Geometry: final body of the model. Coordinates: model frame, mm. Round coordinates to 2 decimals unless told otherwise and drop trailing zeros. Write each loop counter-clockwise with the first axis right and the second up, starting at its lowest first coordinate (ties: lowest second). Pieces come first, ordered by that corner, then holes. Notation, with made-up numbers: (34.25, 79) - (59.25, 79) arc R13 ccw to (59.25, 96) - close; hole circle Ø10 at (68.5, 13.5). An arc over 180 degrees is marked (long way). Write each question's results on one line, items separated by ' | '.
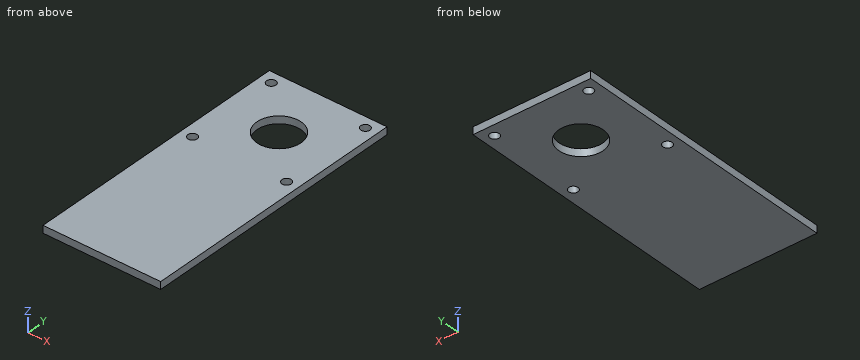
from build123d import *

# Parameters (mm, degrees)
SKETCH2_W           = 50.8
SKETCH2_H           = 50.8
SKETCH2_R           = 2
SKETCH2_R_2         = 9.525
BOSS_EXTRUDE1_DEPTH = 3.175
SKETCH3_W           = 50.8
SKETCH3_H           = 3.175
BOSS_EXTRUDE2_DEPTH = 66.04


with BuildPart() as part:
    # Sketch2 → Boss-Extrude1 (new body)
    with BuildSketch(Plane.XY):
        with Locations((25.4, 25.4)):
            Rectangle(SKETCH2_W, SKETCH2_H)
        with Locations((5.08, 45.72)):
            Circle(SKETCH2_R, mode=Mode.SUBTRACT)
        with Locations((45.72, 45.72)):
            Circle(SKETCH2_R, mode=Mode.SUBTRACT)
        with Locations((45.72, 5.08)):
            Circle(SKETCH2_R, mode=Mode.SUBTRACT)
        with Locations((5.08, 5.08)):
            Circle(SKETCH2_R, mode=Mode.SUBTRACT)
        with Locations((25.4, 25.4)):
            Circle(SKETCH2_R_2, mode=Mode.SUBTRACT)
    extrude(amount=BOSS_EXTRUDE1_DEPTH)

    # Sketch3 → Boss-Extrude2 (add)
    with BuildSketch(Plane.XZ):
        with Locations((25.4, 1.5875)):
            Rectangle(SKETCH3_W, SKETCH3_H)
    extrude(amount=BOSS_EXTRUDE2_DEPTH)


solid = part.part
Q1. Section query B-B, the plane z = 1.8. Return loops of the section in (x, y) (3 decimals).
Answer block:
outline: (0, -66.04) - (50.8, -66.04) - (50.8, 50.8) - (0, 50.8) - close; hole circle Ø4 at (5.08, 5.08); hole circle Ø4 at (5.08, 45.72); hole circle Ø19.05 at (25.4, 25.4); hole circle Ø4 at (45.72, 5.08); hole circle Ø4 at (45.72, 45.72)
Q2. Ray query, line 1 along Y through (x, z) = (45.72, 2.15); line 2 along Y through (x, z) = (25.4, 1.75) (3 decimals); line 3 along X through (y, z) = (30.5, 1.5). Return the intervals inside material, ascending.
Answer block:
line 1: -66.04 to 3.08, 7.08 to 43.72, 47.72 to 50.8 | line 2: -66.04 to 15.875, 34.925 to 50.8 | line 3: 0 to 17.36, 33.44 to 50.8
Q3. Section query A-A, the plane y = 25.4. Return loops of the section in (x, z) (3 decimals), plus the area to 3 significant figures.
Answer block:
outline: (0, 0) - (15.875, 0) - (15.875, 3.175) - (0, 3.175) - close; (34.925, 0) - (50.8, 0) - (50.8, 3.175) - (34.925, 3.175) - close | area: 101 mm2
Q4. Section query D-D, the plane y = 5.08. Return loops of the section in (x, z) (3 decimals).
Answer block:
outline: (0, 0) - (3.08, 0) - (3.08, 3.175) - (0, 3.175) - close; (7.08, 0) - (43.72, 0) - (43.72, 3.175) - (7.08, 3.175) - close; (47.72, 0) - (50.8, 0) - (50.8, 3.175) - (47.72, 3.175) - close
Q5. Section query C-C, the plane x = 45.72. Return loops of the section in (y, z) (3 decimals), plus the area to 3 significant figures.
Answer block:
outline: (-66.04, 0) - (3.08, 0) - (3.08, 3.175) - (-66.04, 3.175) - close; (7.08, 0) - (43.72, 0) - (43.72, 3.175) - (7.08, 3.175) - close; (47.72, 0) - (50.8, 0) - (50.8, 3.175) - (47.72, 3.175) - close | area: 346 mm2
